The listing builds one solid part. Answer for the finished solid, in the listing's coordinates (mm). A direction names the side the tool comes from. Round coordinates to 2 decimals unless told otherwise and drop trailing zeros. Write each loop counter-clockwise with the first axis right and the second up, starting at its lowest first coordinate (ties: lowest second). Pieces come first, ordered by that corner, then holes. Notation, with made-up numbers: (-28, 62.5) - (7, 62.5) arc R29 ccw to (7, 91.5) - close; hole circle Ø1 at (-4, -22). An arc over 180 degrees is marked (long way). Return JSON: item names as keys, results as strings. Group by question number.
from build123d import *

# Parameters (mm, degrees)
BOSS_EXTRUDE1_DEPTH        = 19.3
POT_START                  = -4
POT_INSERT_DEPTH           = 2.5
POT_START_2                = 4
SKETCH6_R                  = 2.75
POT_HOLE_DEPTH             = 40.387513448
SKETCH8_R                  = 2.25
BOSS_EXTRUDE2_DEPTH        = 3
BOSS_EXTRUDE4_START        = 19.3
SKETCH18_R                 = 3
BOSS_EXTRUDE4_DEPTH        = 0.25
BOSS_EXTRUDE3_START        = -0.25
SKETCH17_R                 = 3
BOSS_EXTRUDE3_DEPTH        = 0.25
ABDUCTION_START            = -4
ABDUCTION_CURVE_DEPTH      = 8
ABDUCTION_START_2          = 11
SKETCH13_R                 = 1.75
ABDUCTION_CABLE_HOLE_DEPTH = 9
FLEX_EXTEND_CURVE_DEPTH    = 36.524479064
CUT_EXTRUDE1_START         = -1.5
SKETCH15_W                 = 9
SKETCH15_H                 = 4
CUT_EXTRUDE1_DEPTH         = 4.5
SKETCH16_R                 = 1.25
CUT_EXTRUDE2_DEPTH         = 38.259745213


# Read off the part's stored shape, not the designer's step: Abduction Curve
with BuildPart() as part:
    # Sketch1 → Boss-Extrude1 (new body)
    with BuildSketch(Plane.XY):
        Polygon((1.390238312, 4), (1.390238312, -4), (18.390238312, -4), (29.390238312, -4), (29.390238312, 4), align=None)
    extrude(amount=BOSS_EXTRUDE1_DEPTH)

    # Sketch5 → Pot Insert (cut)
    with BuildSketch(Plane(origin=(0, 0, 0), x_dir=(1, 0, 0), z_dir=(0, 1, 0)).offset(POT_START)):
        Polygon((23.890238312, -11.15), (22.390238312, -14.15), (22.390238312, -15.15), (18.390238312, -15.15), (14.140238312, -15.15), (14.140238312, -14.15), (8.890238312, -14.15), (1.390238312, -14.15), (1.390238312, -9.15), (1.390238312, -5.15), (8.890238312, -5.15), (14.140238312, -5.15), (14.140238312, -4.15), (18.390238312, -4.15), (22.390238312, -4.15), (22.390238312, -5.15), (23.890238312, -8.15), align=None)
    extrude(amount=POT_INSERT_DEPTH, mode=Mode.SUBTRACT)

    # Sketch6 → Pot Hole (cut, through all)
    with BuildSketch(Plane(origin=(0, 0, 0), x_dir=(1, 0, 0), z_dir=(0, 1, 0)).offset(POT_START_2)):
        with Locations(Location((18.390238312, -9.65, 0), (0, 0, 270))):
            Circle(SKETCH6_R)
    extrude(amount=-POT_HOLE_DEPTH, mode=Mode.SUBTRACT)

    # Sketch8 → Boss-Extrude2 (add)
    with BuildSketch(Plane.XY):
        with Locations((18.390238312, 0)):
            Circle(SKETCH8_R)
    extrude(amount=-BOSS_EXTRUDE2_DEPTH)

    # Sketch18 → Boss-Extrude4 (add)
    with BuildSketch(Plane.XY.offset(BOSS_EXTRUDE4_START)):
        with Locations((18.390238312, 0)):
            Circle(SKETCH18_R)
    extrude(amount=BOSS_EXTRUDE4_DEPTH)

    # Sketch17 → Boss-Extrude3 (add)
    with BuildSketch(Plane.XY.offset(BOSS_EXTRUDE3_START)):
        with Locations((18.390238312, 0)):
            Circle(SKETCH17_R)
    extrude(amount=BOSS_EXTRUDE3_DEPTH)

    # Abduction Curve outline → Abduction Curve (cut)
    with BuildSketch(Plane(origin=(0, 0, 0), x_dir=(1, 0, 0), z_dir=(0, 1, 0)).offset(ABDUCTION_START)):
        with BuildLine():
            Line((6.906445385, 0), (1.390238312, 0))
            Line((1.390238312, 0), (1.390238312, -19.3))
            Line((1.390238312, -19.3), (6.906445385, -19.3))
            ThreePointArc((6.906445385, -19.3), (3.390238312, -9.65), (6.906445385, 0))
        make_face()
    extrude(amount=ABDUCTION_CURVE_DEPTH, mode=Mode.SUBTRACT)

    # Sketch13 → Abduction Cable Hole (cut)
    with BuildSketch(Plane.XY.offset(ABDUCTION_START_2)):
        with Locations(Location((18.390238312, 0, 0), (0, 0, 238.997280866))):
            Circle(SKETCH13_R)
    extrude(amount=ABDUCTION_CABLE_HOLE_DEPTH, mode=Mode.SUBTRACT)

    # Sketch14 → Flex-Extend Curve (cut, through all)
    with BuildSketch(Plane.XY):
        with BuildLine():
            Line((29.390238312, 4), (26.046457833, 4))
            ThreePointArc((26.046457833, 4), (28.520661701, 0.335345081), (29.390238312, -4))
            Line((29.390238312, -4), (29.390238312, 4))
        make_face()
    extrude(amount=FLEX_EXTEND_CURVE_DEPTH, mode=Mode.SUBTRACT)

    # Sketch15 → Cut-Extrude1 (cut)
    with BuildSketch(Plane(origin=(0, 0, 0), x_dir=(1, 0, 0), z_dir=(0, 1, 0)).offset(CUT_EXTRUDE1_START)):
        with Locations((13.890238312, -9.65)):
            Rectangle(SKETCH15_W, SKETCH15_H)
    extrude(amount=CUT_EXTRUDE1_DEPTH, mode=Mode.SUBTRACT)

    # Sketch16 → Cut-Extrude2 (cut, through all)
    with BuildSketch(Plane(origin=(0, 0, -3), x_dir=(-1, 0, 0), z_dir=(0, 0, -1))):
        with Locations((-18.390238312, 0)):
            Circle(SKETCH16_R)
    extrude(amount=-CUT_EXTRUDE2_DEPTH, mode=Mode.SUBTRACT)


solid = part.part
(1) Find section A-A (z = 9.65). Write down the section's boundary in (x, y).
(2) Consider line 1 (Z direction, x = 15, y = -2); line 2 (Z direction, x = 15.25, y = -1.25); line 3 (Y direction, x = 16, z = 14). Determine where each line is inside the solid, lowest interval first.
(3) Flat-ended cylindrical pins translate along their axes: pin 1 (4.5 mm diameter, centred on y = 1.5, z = 10, fed in from +X); pin 2 (2 mm diameter, centred on x = 18.39, y = 0, fed in from +Z); pin 3 (3 mm diameter, centred on x = 14, z = 9, fed in from -Y); pin 4 (4 mm diameter, centred on y = -0.5, z = 11.5, fed in from +X). Find the tip coordinate at first contact, or state that the pin passes through.
(4) Find section C-C (x = 12). Write down the section's boundary in (y, z), plus the area to 3 significant figures.
(5) For faces 3 (the flat face through (23.15, -2.77, 12.63)), 4 (the flat face through (21, 0, -0.25)), 5 (the flat face through (14.14, -3, 5)), determine the directions among +Z, -Z, +X, -X, +Y, -Y from which every point of the face is accessible in a straight line to the end or side of a thin tool.
(6) Determine the mould class of faces 1 (the cylindrical face through (18.19, 1.74, 15.61)), 2 (the flat face through (14.14, -3, 15)) for opening direction Y: +Y half, -Y half, draft (parallel to the pull), parting line (faces both ways), or undercut.
(7) Find section B-B (y = 0). Write down the section's boundary in (x, z).
(8) Find section D-D (y = -3.5). Write down the section's boundary in (x, z).
Check sheet entries:
{
 "1": {"outline": "(3.39, -1.5) - (9.39, -1.5) - (9.39, 3) - (15.64, 3) - (15.64, 4) - (3.39, 4) - close; (21.14, -1.5) - (23.89, -1.5) - (23.89, -4) - (29.39, -4) arc R11.24 ccw to (26.05, 4) - (21.14, 4) - close"},
 "2": {"line 1": "z = 0 to 4.15, 15.15 to 19.3", "line 2": "z = 0 to 7.65, 11.65 to 19.3", "line 3": "y = -1.5 to 4"},
 "3": {"pin 1": "stops at x = 28.91", "pin 2": "passes through", "pin 3": "stops at y = -1.5", "pin 4": "stops at x = 29.29"},
 "4": {"outline": "(-4, 0) - (4, 0) - (4, 19.3) - (-4, 19.3) - (-4, 14.15) - (-1.5, 14.15) - (-1.5, 11.65) - (3, 11.65) - (3, 7.65) - (-1.5, 7.65) - (-1.5, 5.15) - (-4, 5.15) - close", "area": "114 mm^2"},
 "5": {"face 3": "-X, -Y", "face 4": "-Z", "face 5": "-Y"},
 "6": {"face 1": "undercut", "face 2": "draft"},
 "7": {"outline": "(6.91, 0) - (15.39, 0) - (15.39, -0.25) - (16.14, -0.25) - (16.14, -3) - (17.14, -3) - (17.14, 7.2) arc R2.75 cw to (16.5, 7.65) - (9.39, 7.65) - (9.39, 11.65) - (16.5, 11.65) arc R2.75 cw to (16.64, 11.77) - (16.64, 19.55) - (15.39, 19.55) - (15.39, 19.3) - (6.91, 19.3) arc R15 ccw to start; (19.64, -3) - (20.64, -3) - (20.64, -0.25) - (21.39, -0.25) - (21.39, 0) - (28.65, 0) - (28.65, 19.3) - (21.39, 19.3) - (21.39, 19.55) - (20.14, 19.55) - (20.14, 11.77) arc R2.75 cw to (19.64, 7.2) - close"},
 "8": {"outline": "(4.08, 5.15) arc R15 ccw to (6.91, 0) - (29.38, 0) - (29.38, 19.3) - (6.91, 19.3) arc R15 ccw to (4.08, 14.15) - (14.14, 14.15) - (14.14, 15.15) - (22.39, 15.15) - (22.39, 14.15) - (23.89, 11.15) - (23.89, 8.15) - (22.39, 5.15) - (22.39, 4.15) - (14.14, 4.15) - (14.14, 5.15) - close"}
}
